from build123d import *

# Parameters (mm, degrees)
SKETCH2_R                        = 21.59
SKETCH2_R_2                      = 10.922
BOSS_EXTRUDE1_DEPTH              = 38.1
CUT_EXTRUDE1_REACH               = 50.825
SKETCH3_W                        = 21.59
SKETCH3_H                        = 1.5875
CUT_EXTRUDE2_REACH               = 50.825
SKETCH4_R                        = 3.0226
CUT_EXTRUDE3_REACH               = 50.825
TAP_DRILL_FOR_M3X0_5_TAP1_D      = 2.5
TAP_DRILL_FOR_M3X0_5_TAP1_DEPTH  = 4.572
TAP_DRILL_FOR_M3X0_5_TAP1_TIP    = 0.751075774
CUT_EXTRUDE4_REACH               = 62.615
CUT_EXTRUDE4_END_RADIUS          = 3.0226
SKETCH8_R                        = 1.650000002
TAP_DRILL_FOR_M4X0_7_TAP1_REACH  = 54.19
TAP_DRILL_FOR_M4X0_7_TAP1_BORE_R = 1.65


with BuildPart() as part:
    # Sketch2 → Boss-Extrude1 (new body)
    with BuildSketch(Plane(origin=(0, 0, 0), x_dir=(1, 0, 0), z_dir=(0, 1, 0))):
        with Locations(Location((0, 0, 0), (0, 0, 90))):
            Circle(SKETCH2_R)
        with Locations(Location((0, 0, 0), (0, 0, 90))):
            Circle(SKETCH2_R_2, mode=Mode.SUBTRACT)
    extrude(amount=BOSS_EXTRUDE1_DEPTH)

    # Sketch3 → Cut-Extrude1 (cut, up to next)
    with BuildSketch(Plane(origin=(0, 38.1, 0), x_dir=(1, 0, 0), z_dir=(0, 1, 0)), mode=Mode.PRIVATE) as cut_extrude1_sk1:
        with Locations((-10.795, 0)):
            Rectangle(SKETCH3_W, SKETCH3_H)
    cut_extrude1_tool1 = extrude(cut_extrude1_sk1.sketch, amount=-CUT_EXTRUDE1_REACH, mode=Mode.PRIVATE) & part.part
    add(cut_extrude1_tool1.solids().sort_by_distance((-10.795, 38.1, 0))[0], mode=Mode.SUBTRACT)

    # Sketch4 → Cut-Extrude2 (cut, up to next)
    with BuildSketch(Plane(origin=(0, 38.1, 0), x_dir=(1, 0, 0), z_dir=(0, 1, 0)), mode=Mode.PRIVATE) as cut_extrude2_sk1:
        with Locations(Location((0, -16.256, 0), (0, 0, 270))):
            Circle(SKETCH4_R)
    cut_extrude2_tool1 = extrude(cut_extrude2_sk1.sketch, amount=-CUT_EXTRUDE2_REACH, mode=Mode.PRIVATE) & part.part
    add(cut_extrude2_tool1.solids().sort_by_distance((0, 38.1, 16.256))[0], mode=Mode.SUBTRACT)

    # Sketch5 → Cut-Extrude3 (cut, up to next)
    with BuildSketch(Plane(origin=(0, 38.1, 0), x_dir=(1, 0, 0), z_dir=(0, 1, 0)), mode=Mode.PRIVATE) as cut_extrude3_sk1:
        with BuildLine():
            Line((7.295594561, 20.32), (-7.295594561, 20.32))
            ThreePointArc((-7.295594561, 20.32), (0, 21.59), (7.295594561, 20.32))
        make_face()
    cut_extrude3_tool1 = extrude(cut_extrude3_sk1.sketch, amount=-CUT_EXTRUDE3_REACH, mode=Mode.PRIVATE) & part.part
    add(cut_extrude3_tool1.solids().sort_by_distance((0, 38.1, -20.829303))[0], mode=Mode.SUBTRACT)

    # Tap Drill for M3x0.5 Tap1
    with Locations(Plane(origin=(0, 19.05, -20.32), x_dir=(-1, 0, 0), z_dir=(0, 0, -1))):
        with Locations((0, 0)):
            Hole(TAP_DRILL_FOR_M3X0_5_TAP1_D / 2, depth=TAP_DRILL_FOR_M3X0_5_TAP1_DEPTH)
            with Locations((0, 0, -(TAP_DRILL_FOR_M3X0_5_TAP1_DEPTH + TAP_DRILL_FOR_M3X0_5_TAP1_TIP / 2))):  # 118° drill point
                Cone(0, TAP_DRILL_FOR_M3X0_5_TAP1_D / 2, TAP_DRILL_FOR_M3X0_5_TAP1_TIP, mode=Mode.SUBTRACT)

    # Cut-Extrude4: up to this cylinder (the profile starts outside it)
    cut_extrude4_end = Plane(origin=(0, 19.609114, 16.256), z_dir=(0, 1, 0)) * Cylinder(CUT_EXTRUDE4_END_RADIUS, 132.2752, mode=Mode.PRIVATE)
    # Sketch8 → Cut-Extrude4 (cut, up to the surface)
    with BuildSketch(Plane.XY.offset(21.59), mode=Mode.PRIVATE) as cut_extrude4_sk1:
        with Locations((0, 19.609113622)):
            Circle(SKETCH8_R)
    cut_extrude4_tool1 = extrude(cut_extrude4_sk1.sketch, amount=-CUT_EXTRUDE4_REACH, mode=Mode.PRIVATE) - cut_extrude4_end
    add(cut_extrude4_tool1.solids().sort_by_distance((0, 19.609114, 21.59))[0], mode=Mode.SUBTRACT)

    # Tap Drill for M4x0.7 Tap1 bore (on position points) → Tap Drill for M4x0.7 Tap1 (cut, up to next)
    with BuildSketch(Plane(origin=(-16.234261615, 29.109235595, 0.79375), x_dir=(-1, 0, 0), z_dir=(0, 0, -1)), mode=Mode.PRIVATE) as tap_drill_for_m4x0_7_tap1_sk1:
        Circle(TAP_DRILL_FOR_M4X0_7_TAP1_BORE_R)
    tap_drill_for_m4x0_7_tap1_tool1 = extrude(tap_drill_for_m4x0_7_tap1_sk1.sketch, amount=-TAP_DRILL_FOR_M4X0_7_TAP1_REACH, mode=Mode.PRIVATE) & part.part
    # Tap Drill for M4x0.7 Tap1 bore (on position points) → Tap Drill for M4x0.7 Tap1 (cut, up to next)
    with BuildSketch(Plane(origin=(-16.234261615, 29.109235595, 0.79375), x_dir=(-1, 0, 0), z_dir=(0, 0, -1)), mode=Mode.PRIVATE) as tap_drill_for_m4x0_7_tap1_sk2:
        with Locations((0, -20.205281104)):
            Circle(TAP_DRILL_FOR_M4X0_7_TAP1_BORE_R)
    tap_drill_for_m4x0_7_tap1_tool2 = extrude(tap_drill_for_m4x0_7_tap1_sk2.sketch, amount=-TAP_DRILL_FOR_M4X0_7_TAP1_REACH, mode=Mode.PRIVATE) & part.part
    add(tap_drill_for_m4x0_7_tap1_tool1.solids().sort_by_distance((-16.234262, 29.109236, 0.79375))[0], mode=Mode.SUBTRACT)
    add(tap_drill_for_m4x0_7_tap1_tool2.solids().sort_by_distance((-16.234262, 8.903954, 0.79375))[0], mode=Mode.SUBTRACT)


solid = part.part
Design review of the part built by this model. Coordinates are the model's own, in mm. A direction names the side the tool comes from. Round coordinates to 2 decimals unless told otherwise and drop trailing zeros. Loops run counter-clockwise (first coordinate to the right, second up) from the corner with the lowest first, then second, coordinate; pieces in that order, holes last. Notation, with made-up numbers: (53, 43) - (102, 43) arc R14 ccw to (102, 56) - close; hole circle Ø2 at (-31, 33). An arc over 180 degrees is marked (long way). One line per question, with ' | ' between items.
1. We need section A-A, the plane z = 8.5. State the section outline as (x, y) points.
Results are:
outline: (-19.85, 0) - (-6.86, 0) - (-6.86, 38.1) - (-19.85, 38.1) - close; (6.86, 0) - (19.85, 0) - (19.85, 38.1) - (6.86, 38.1) - close; hole circle Ø3.3 at (-16.23, 8.9); hole circle Ø3.3 at (-16.23, 29.11)
2. We need section D-D, the plane z = -8. State the section outline as (x, y) points.
Results are:
outline: (-20.05, 0) - (-7.44, 0) - (-7.44, 38.1) - (-20.05, 38.1) - close; (7.44, 0) - (20.05, 0) - (20.05, 38.1) - (7.44, 38.1) - close
3. For faces 1 (the face through (5, 0, 10)), 2 (the face through (-14.586, 8.977, 8.251)), 3 (the face through (-0.27, 17.83, -18)), 4 (the face through (-16, 19, 0.794)), list the 3-axis set-ups (+Z, -Z, +X, -X, +Y, -Y) from which the entire face can be reached by the end or side of a thin tool; tool diameter is ignored.
Results are:
face 1: +Z, -Z, +X, -X, -Y | face 2: +Z | face 3: -Z | face 4: -X, +Y, -Y
4. Clearance check with flat-ended pins moving along their axes: P1, Ø1, axis at x = -15.5, y = 26, coming from the +Z side; P2, Ø3, axis at x = 0, y = 19.61, coming from the +Z side; P3, Ø4, axis at y = 32.5, z = 3.5, coming from the -X side. State where each tip first meets the part, or that it passes through.
Results are:
P1: stops at z = 15.53 | P2: stops at z = 13.63 | P3: stops at x = -21.54
5. We need section C-C, the plane z = 14. State the section outline as (x, y) points, and give its area (3 significant figures).
Results are:
outline: (-16.44, 0) - (-2.01, 0) - (-2.01, 38.1) - (-16.44, 38.1) - (-16.44, 30.75) arc R1.65 cw (long way) to (-16.44, 27.47) - (-16.44, 10.54) arc R1.65 cw (long way) to (-16.44, 7.27) - close; (2.01, 0) - (16.44, 0) - (16.44, 38.1) - (2.01, 38.1) - close | area: 1,090 mm²
6. For L1, parallel to Y at x = 0, z = -17; L2, parallel to Z at x = -1, y = 23; L3, parallel to X at y = 24, z = 1, list the stretches that pass through material, from the lowest coordinate up. Write a range as [from, to].
Results are:
L1: y = [0, 17.8], [20.3, 38.1] | L2: z = [-20.32, -10.88], [10.88, 13.4], [19.11, 21.57] | L3: x = [-21.57, -10.88], [10.88, 21.57]
7. We need section B-B, the plane y = 13.5. State the section outline as (x, z) points.
Results are:
outline: (-21.58, -0.79) arc R21.59 ccw to (-7.3, -20.32) - (7.3, -20.32) arc R21.59 ccw (long way) to (-21.58, 0.79) - (-10.89, 0.79) arc R10.92 cw (long way) to (-10.89, -0.79) - close; hole circle Ø6.05 at (0, 16.26)
8. Draft analysis for pull direction Z (two halves, no side actions). For faces 5 (the face through (12.211, 18.783, 17.805)), 6 (the face through (-17.32, 18.78, -12.89)), 7 (the face through (5, 38.1, 10)), 8 (the face through (0.133, 19.317, 13.236)), state which applies: released by +Z, released by -Z, zero draft, split by the parting line, or undercut.
Results are:
face 5: split by the parting line | face 6: released by -Z | face 7: zero draft | face 8: undercut
